Autodesk Inventor part; units mm, degrees
ref_plane "YZ Plane" through (0, 0, 0) normal (1, 0, 0) x (0, 1, 0)
ref_plane "XZ Plane" through (0, 0, 0) normal (0, 1, 0) x (-1, 0, 0)
ref_plane "XY Plane" through (0, 0, 0) normal (0, 0, 1) x (1, 0, 0)
sketch "Sketch1" plane through (0, 0, 0) normal (0, 0, 1) x (1, 0, 0)
  line L0 (-2, 0) -> (2, 0)
  arc A0 (8.313, 9.4417) -> (-8.313, 9.4417) centre (0, 15) ccw
  line L1 (-2, 0) -> (-8.313, 9.4417)
  line L2 (2, 0) -> (8.313, 9.4417)
  line L3 (0, 0) -> (0, 7.2801) construction
  point P0 (0, 3.6401)
  dimension "d0" = 20
  dimension "d1" = 4
  dimension "d2" = 15
extrude "Extrusion1" add sketch "Sketch1" along normal mid plane 3
sketch "Sketch2" plane through (0, 0, 1.5) normal (0, 0, 1) x (1, 0, 0)
  circle A0 centre (0, 15) radius 9
  arc A1 (8.313, 9.4417) -> (-8.313, 9.4417) centre (0, 15) ccw
  point P0 (0, 0)
  dimension "d5" = 18
extrude "Extrusion2" cut sketch "Sketch2" against normal blind 3
sketch "Sketch3" plane through (-2, 0, 1.5) normal (0, -1, 0) x (1, 0, 0)
  circle A0 centre (2, -1.5) radius 1.25
  dimension "d8" = 2.5
extrude "Extrusion3" cut sketch "Sketch3" against normal up to surface
properties part number "21"
Can you work these out from the model? Positions are in its coordinate system, mm. Give positions to 0.01 mm unless a question says otherwise; leave off trailing zeros. Order: outer loops, then holes, each group sorted by start corner. A loop starts at its lowest first (then second) coordinate and runs counter-clockwise, first axis right, second up. Notation, with made-up numbers: M -36.5,83 L -28.5,83 A8 ccw -28.5,87 Z; hole C -31.75,-22 d4. An arc over 180 degrees is marked long. Use a Markdown table: item, result. Add a question column.
Item 1: Will these pins go through, and if not, where does the flat tip stop? pin 1 (2 mm diameter, centred on x = -5.5, y = 12, fed in from +Z); pin 2 (1.5 mm diameter, centred on y = 11.5, z = -0.5, fed in from -X).
Item 2: Suppose I cut it at D-D (x = -6.5). List the corners of the cut face in (y, z) for me.
Item 3: Suppose I cut it at A-A (x = 0). List the corners of the cut face in (y, z) for me, then the cut area to 3 significant figures.
Item 4: If I drill on L1, parallel to Z at x = 0, y = 3.25; L2, parallel to Y at x = 0, z = -0.35; L3, parallel to Y at x = 2.5, z = -0.75, over which ranges is the centre line in solid material (lowest first)? Write a range as [from, to].
Item 5: We'd pull the mould along Z, two halves only. Please class faces 1 (the flat face through (-2, 6, -1.5)), 2 (the cylindrical face through (0, 25, 0)), 3 (the flat face through (-2, 6, 1.5)), 4 (the cylindrical face through (1.19, 3, 0.38)): +Z half, -Z half, draft (parallel to the pull), parting line (faces both ways), or undercut.
Item 6: Suppose I cut it at C-C (z = 0). List the corners of the cut face in (x, y) for me.
Item 7: Suppose I cut it at B-B (y = 15). List the corners of the cut face in (x, z) for me, then the cut area to 3 significant figures.
Answer sheet:
| question | item | result |
|---|---|---|
| 1 | pin 1 | passes through |
| 1 | pin 2 | stops at x = -9.61 |
| 2 | outline | M 6.73,-1.5 L 8.78,-1.5 L 8.78,1.5 L 6.73,1.5 Z; M 21.22,-1.5 L 22.6,-1.5 L 22.6,1.5 L 21.22,1.5 Z |
| 3 | outline | M 0,-1.5 L 6,-1.5 L 6,-1.25 L 0,-1.25 Z; M 0,1.25 L 6,1.25 L 6,1.5 L 0,1.5 Z; M 24,-1.5 L 25,-1.5 L 25,1.5 L 24,1.5 Z |
| 3 | area | 6.00 mm² |
| 4 | L1 | z = [-1.5, -1.25], [1.25, 1.5] |
| 4 | L2 | y = [24, 25] |
| 4 | L3 | y = [0.75, 6.35], [23.65, 24.68] |
| 5 | face 1 | -Z half |
| 5 | face 2 | draft |
| 5 | face 3 | +Z half |
| 5 | face 4 | undercut |
| 6 | outline | M -8.31,9.44 L -2,0 L -1.25,0 L -1.25,6.09 A9 cw long 1.25,6.09 L 1.25,0 L 2,0 L 8.31,9.44 A10 ccw long Z |
| 7 | outline | M -10,-1.5 L -9,-1.5 L -9,1.5 L -10,1.5 Z; M 9,-1.5 L 10,-1.5 L 10,1.5 L 9,1.5 Z |
| 7 | area | 6.00 mm² |
